Verification items for the finished model (mm, model axes). A direction names the side the tool comes from. Round coordinates to 2 decimals unless told otherwise and drop trailing zeros. Order: outer loops, then holes, each group sorted by start corner. A loop starts at its lowest first (then second) coordinate and runs counter-clockwise, first axis right, second up. Notation, with made-up numbers: M 29,81.5 L 58,81.5 A21 ccw 58,105.5 Z; hole C -30,32 d11. An arc over 180 degrees is marked long. Answer as a JSON object with one key per item and string values. Group by question number.
```python
from build123d import *

# Parameters (mm, degrees)
SKETCH1_W           = 120
SKETCH1_H           = 50
BOSS_EXTRUDE1_DEPTH = 10
SKETCH2_R           = 1.5
CUT_EXTRUDE1_DEPTH  = 11
SKETCH3_R           = 2.5
CUT_EXTRUDE2_DEPTH  = 11
SKETCH4_R           = 4.25
CUT_EXTRUDE3_DEPTH  = 5


with BuildPart() as part:
    # Sketch1 → Boss-Extrude1 (new body)
    with BuildSketch(Plane(origin=(0, 0, 0), x_dir=(1, 0, 0), z_dir=(0, 1, 0))):
        Rectangle(SKETCH1_W, SKETCH1_H)
    extrude(amount=BOSS_EXTRUDE1_DEPTH)

    # Sketch2 → Cut-Extrude1 (cut, through all)
    with BuildSketch(Plane(origin=(0, 10, 0), x_dir=(1, 0, 0), z_dir=(0, 1, 0))):
        with Locations((28, -12)):
            Circle(SKETCH2_R)
        with Locations((28, 12)):
            Circle(SKETCH2_R)
        with Locations((46, -12)):
            Circle(SKETCH2_R)
        with Locations((46, 12)):
            Circle(SKETCH2_R)
        with Locations((-46, -12)):
            Circle(SKETCH2_R)
        with Locations((-46, 12)):
            Circle(SKETCH2_R)
        with Locations((-28, -12)):
            Circle(SKETCH2_R)
        with Locations((-28, 12)):
            Circle(SKETCH2_R)
    extrude(amount=-CUT_EXTRUDE1_DEPTH, mode=Mode.SUBTRACT)

    # Sketch3 → Cut-Extrude2 (cut, through all)
    with BuildSketch(Plane.XZ):
        Circle(SKETCH3_R)
        with Locations((30, 0)):
            Circle(SKETCH3_R)
        with Locations((-30, 0)):
            Circle(SKETCH3_R)
    extrude(amount=-CUT_EXTRUDE2_DEPTH, mode=Mode.SUBTRACT)

    # Sketch4 → Cut-Extrude3 (cut)
    with BuildSketch(Plane.XZ):
        with Locations((30, 0)):
            Circle(SKETCH4_R)
        Circle(SKETCH4_R)
        with Locations((-30, 0)):
            Circle(SKETCH4_R)
    extrude(amount=-CUT_EXTRUDE3_DEPTH, mode=Mode.SUBTRACT)


solid = part.part
```
Q1. Release check for a two-part mould opening along X. For faces 1 (the face through (-29.5, 5.07, -12.07)), 2 (the face through (26.5, 5.07, 11.93)), 3 (the face through (-60, 5, 0)), 4 (the face through (-1, 10, -6)) record: released by +X, released by -X, zero draft, split by the parting line, or undercut.
Q2. Cross-section at B-B, the plane y = 3. Give the number of separate pieces and of enclosed holes in the cut face, then the cut area to 3 significant figures.
Q3. Thickness scan on line 1 (X direction, y = 1.5, z = -12); line 2 (X direction, y = 2.5, z = -11); line 3 (X direction, y = 0.5, z = -2.5). Record the ranges inside material, lowest first. Write a range as from..to.
Q4. Gauge pin test, flat end, axial feed: pin 1 Ø4 at (x, z) = (30.5, -0.5) entering from -Y. Record the tip position at first contact, or that the pin passes through.
Q5. Cross-section at A-A, the plane z = 0. Record the cut outline in (x, y), then the cut area to 4 significant figures.
Q6. Tool access check on faces 5 (the face through (-1, 5, -25)), 6 (the face through (25.754, 2.465, 0.187)). Record the directions out of +Z, -Z, +X, -X, +Y, -Y that give a thin tool (end or side, any length) a straight path to the whole face; none if there is none.
Conclusion:
{
 "1": {"face 1": "undercut", "face 2": "undercut", "face 3": "released by -X", "face 4": "zero draft"},
 "2": {"separate pieces": "1", "enclosed holes": "11", "area": "5,770 mm2"},
 "3": {"line 1": "-60..-47.5, -44.5..-29.5, -26.5..26.5, 29.5..44.5, 47.5..60", "line 2": "-60..-47.12, -44.88..-29.12, -26.88..26.88, 29.12..44.88, 47.12..60", "line 3": "-60..-33.44, -26.56..-3.44, 3.44..26.56, 33.44..60"},
 "4": {"pin 1": "y = 5"},
 "5": {"outline": "M -60,0 L -34.25,0 L -34.25,5 L -32.5,5 L -32.5,10 L -60,10 Z; M -27.5,5 L -25.75,5 L -25.75,0 L -4.25,0 L -4.25,5 L -2.5,5 L -2.5,10 L -27.5,10 Z; M 2.5,5 L 4.25,5 L 4.25,0 L 25.75,0 L 25.75,5 L 27.5,5 L 27.5,10 L 2.5,10 Z; M 32.5,5 L 34.25,5 L 34.25,0 L 60,0 L 60,10 L 32.5,10 Z", "area": "997.5 mm2"},
 "6": {"face 5": "-Z, +X, -X, +Y, -Y", "face 6": "-Y"}
}
